from build123d import *

# Parameters (mm, degrees)
BOSS_EXTRUDE1_DEPTH = 1.5
CUT_EXTRUDE4_DEPTH  = 0.5
SKETCH3_W           = 8.5
SKETCH3_H           = 6.5
BOSS_EXTRUDE2_DEPTH = 5
SKETCH4_W           = 8.5
SKETCH4_H           = 5.5
CUT_EXTRUDE1_DEPTH  = 4
CUT_EXTRUDE2_DEPTH  = 33
FILLET1_R           = 3
SKETCH6_W           = 5
SKETCH6_H           = 2.5
CUT_EXTRUDE3_DEPTH  = 1.5
BOSS_EXTRUDE4_DEPTH = 3
SKETCH10_R          = 1
BOSS_EXTRUDE5_DEPTH = 2.5
FILLET2_R           = 1


with BuildPart() as part:
    # Sketch2 → Boss-Extrude1 (new body)
    with BuildSketch(Plane(origin=(0, 0, 0), x_dir=(1, 0, 0), z_dir=(0, 1, 0))):
        with BuildLine():
            Line((-61.5, 13.25), (61.5, 13.25))
            Line((61.5, 13.25), (61.5, -13.25))
            ThreePointArc((61.5, -13.25), (61.060660172, -14.310660172), (60, -14.75))
            Line((60, -14.75), (-60, -14.75))
            ThreePointArc((-60, -14.75), (-61.060660172, -14.310660172), (-61.5, -13.25))
            Line((-61.5, -13.25), (-61.5, 13.25))
        make_face()
    extrude(amount=BOSS_EXTRUDE1_DEPTH)

    # Sketch9 → Cut-Extrude4 (cut)
    with BuildSketch(Plane.XZ):
        with BuildLine():
            Line((60, -13.25), (65, -13.25))
            Line((65, -13.25), (65, 18.25))
            Line((65, 18.25), (-65, 18.25))
            Line((-65, 18.25), (-65, -13.25))
            Line((-65, -13.25), (-60, -13.25))
            Line((-60, -13.25), (-60, 12.45))
            ThreePointArc((-60, 12.45), (-59.765685425, 13.015685425), (-59.2, 13.25))
            Line((-59.2, 13.25), (59.2, 13.25))
            ThreePointArc((59.2, 13.25), (59.765685425, 13.015685425), (60, 12.45))
            Line((60, 12.45), (60, -13.25))
        make_face()
    extrude(amount=-CUT_EXTRUDE4_DEPTH, mode=Mode.SUBTRACT)

    # Sketch3 → Boss-Extrude2 (add)
    with BuildSketch(Plane(origin=(0, 1.5, 0), x_dir=(1, 0, 0), z_dir=(0, 1, 0))):
        with Locations((-40.25, -15.5)):
            Rectangle(SKETCH3_W, SKETCH3_H)
    boss_extrude2 = extrude(amount=-BOSS_EXTRUDE2_DEPTH)

    # Sketch4 → Cut-Extrude1 (cut)
    with BuildSketch(Plane(origin=(0, 1.5, 0), x_dir=(1, 0, 0), z_dir=(0, 1, 0))):
        with Locations((-40.25, -16)):
            Rectangle(SKETCH4_W, SKETCH4_H)
    cut_extrude1 = extrude(amount=-CUT_EXTRUDE1_DEPTH, mode=Mode.SUBTRACT)

    # Sketch5 → Cut-Extrude2 (cut, through all)
    with BuildSketch(Plane.XY.offset(18.75)):
        Polygon((-44.5, 0), (-43.5, -3.5), (-44.5, -3.5), align=None)
        Polygon((-36, 0), (-36, -3.5), (-37, -3.5), align=None)
    cut_extrude2 = extrude(amount=-CUT_EXTRUDE2_DEPTH, mode=Mode.SUBTRACT)

    # Mirror1: Boss-Extrude2, Cut-Extrude1, Cut-Extrude2 across plane
    add(boss_extrude2.mirror(Plane(origin=(0, 0, 0), x_dir=(0, 0, 1), z_dir=(1, 0, 0))))
    add(cut_extrude1.mirror(Plane(origin=(0, 0, 0), x_dir=(0, 0, 1), z_dir=(1, 0, 0))), mode=Mode.SUBTRACT)
    add(cut_extrude2.mirror(Plane(origin=(0, 0, 0), x_dir=(0, 0, 1), z_dir=(1, 0, 0))), mode=Mode.SUBTRACT)

    # Fillet1
    fillet1_edges = [part.edges().sort_by_distance(p)[0] for p in [
        (40.25, 0, 12.25),
        (-40.25, 0, 12.25),
    ]]
    fillet(fillet1_edges, radius=FILLET1_R)

    # Sketch6 → Cut-Extrude3 (cut)
    with BuildSketch(Plane(origin=(0, 1.5, 0), x_dir=(1, 0, 0), z_dir=(0, 1, 0))):
        with Locations((-59, 12)):
            Rectangle(SKETCH6_W, SKETCH6_H)
    cut_extrude3 = extrude(amount=-CUT_EXTRUDE3_DEPTH, mode=Mode.SUBTRACT)

    # Sketch7 → Boss-Extrude4 (add)
    with BuildSketch(Plane.ZY.offset(56.5)):
        with BuildLine():
            Line((-10.75, 0), (-10.75, -0.5))
            ThreePointArc((-10.75, -0.5), (-11.068858925, -1.37188366), (-11.047594135, -2.3))
            Line((-11.047594135, -2.3), (-10.75, -3))
            Line((-10.75, -3), (-9.75, -3))
            Line((-9.75, -3), (-9.75, 0))
            Line((-9.75, 0), (-10.75, 0))
        make_face()
    boss_extrude4 = extrude(amount=BOSS_EXTRUDE4_DEPTH)

    # Mirror2: Cut-Extrude3, Boss-Extrude4 across plane
    add(cut_extrude3.mirror(Plane(origin=(0, 0, 0), x_dir=(0, 0, 1), z_dir=(1, 0, 0))), mode=Mode.SUBTRACT)
    add(boss_extrude4.mirror(Plane(origin=(0, 0, 0), x_dir=(0, 0, 1), z_dir=(1, 0, 0))))

    # Sketch10 → Boss-Extrude5 (add)
    with BuildSketch(Plane(origin=(0, 0, 0), x_dir=(-1, 0, 0), z_dir=(0, -1, 0))):
        with Locations((-15, 11.5)):
            Circle(SKETCH10_R)
        with Locations((15, 11.5)):
            Circle(SKETCH10_R)
    extrude(amount=BOSS_EXTRUDE5_DEPTH)

    # Fillet2
    fillet2_edges = [part.edges().sort_by_distance(p)[0] for p in [
        (-58, 0, -9.75),
        (58, 0, -9.75),
    ]]
    fillet(fillet2_edges, radius=FILLET2_R)


solid = part.part
Design review of the part built by this model. Coordinates are the model's own, in mm. A direction names the side the tool comes from. Round coordinates to 2 decimals unless told otherwise and drop trailing zeros. Write each loop counter-clockwise with the first axis right and the second up, starting at its lowest first coordinate (ties: lowest second). Pieces come first, ordered by that corner, then holes. Notation, with made-up numbers: M -35.75,75 L 4.25,75 A24 cw 4.25,86 Z; hole C 44,82.25 d9. An arc over 180 degrees is marked long. One line per item, written item: value. Start each with the question number.
1. Draft analysis for pull direction X (two halves, no side actions). For faces 1 (the face through (-40, -3.5, 15)), 2 (the face through (-43.7, -2.8, 14.4)), 3 (the face through (-15.924, -1.232, -11.117)), state which applies: pulls with the +X half, pulls with the -X half, needs draft (parallel to the pull), parting line crosses it, or undercut.
2. For faces 4 (the face through (-61, 0.5, 8)), 5 (the face through (-40, -2.5, 16)), 6 (the face through (-59.5, -1, -10)), 7 (the face through (36.762, -2.666, 14.726)), list the 3-axis set-ups (+Z, -Z, +X, -X, +Y, -Y) from which the entire face can be reached by the end or side of a thin tool; tool diameter is ignored.
3. Clearance check with flat-ended pins moving along their axes: P1, Ø1.1, axis at y = 1, z = 14, coming from the +X side; P2, Ø13.5, axis at x = -51.5, z = 7, coming from the -Y side; P3, Ø1.2, axis at y = 0.5, z = -12, coming from the -X side. State where each tip first meets the part, or that it passes through.
4. Take a section at A-A on z = 4.5. State the section outline as (x, y) points.
5. Take a section at B-B on x = -20. State the section outline as (y, z) points, then the cut area to 4 significant figures.
6. To check wall thickness, follow probe 1 along Y at (x, z) = (-37.5, 2); probe 2 along X at (y, z) = (0.7, 14); probe 3 along X at (y, z) = (0.1, -1.5). State the ranges of each line that lie inside material, in increasing order. Write a range as from..to.
Computed:
1. face 1: needs draft
1. face 2: pulls with the -X half
1. face 3: undercut
2. face 4: +Z, -X, -Y
2. face 5: +Z, +X, -X, +Y
2. face 6: +Z, -Z, -X, -Y
2. face 7: +Z, -Z, -Y
3. P1: stops at x = 61.49
3. P2: stops at y = 0
3. P3: stops at x = -56.5
4. outline: M -61.5,0.5 L -60,0.5 L -60,0 L 60,0 L 60,0.5 L 61.5,0.5 L 61.5,1.5 L -61.5,1.5 Z
5. outline: M 0,-13.25 L 1.5,-13.25 L 1.5,14.75 L 0.5,14.75 L 0.5,13.25 L 0,13.25 Z
5. area: 41.25 mm²
6. probe 1: y = 0..1.5
6. probe 2: x = -61.3..-44.5, -36..36, 44.5..61.3
6. probe 3: x = -60..60
